Here's how the part is built. I have some questions about the finished solid (model axes, mm). A direction names the side the tool comes from. Coordinates: 2 decimals unless noted, no trailing zeros. Order: outer loops, then holes, each group sorted by start corner. A loop starts at its lowest first (then second) coordinate and runs counter-clockwise, first axis right, second up. Notation, with made-up numbers: (-3.5, 84.5) - (24.5, 84.5) arc R5 ccw to (24.5, 90.5) - close; hole circle Ø5 at (18, 15.5). An arc over 180 degrees is marked (long way). Use one line per item in the form item = value. Start each with the question number.
from build123d import *

# Parameters (mm, degrees)
SKETCH1_R                      = 16
SKETCH1_R_2                    = 4
BOSS_EXTRUDE1_DEPTH            = 2
SKETCH2_R                      = 8
SKETCH2_R_2                    = 4
BOSS_EXTRUDE2_DEPTH            = 11
M4_CLEARANCE_HOLE1_D           = 4.5
M4_CLEARANCE_HOLE1_DEPTH       = 13
M4_CLEARANCE_HOLE1_CSINK_D     = 4.55
M4_CLEARANCE_HOLE1_CSINK_ANGLE = 90
M4_CLEARANCE_HOLE1_TIP         = 1.351936393


with BuildPart() as part:
    # Sketch1 → Boss-Extrude1 (new body)
    with BuildSketch(Plane(origin=(0, 0, 0), x_dir=(1, 0, 0), z_dir=(0, 1, 0))):
        Circle(SKETCH1_R)
        Circle(SKETCH1_R_2, mode=Mode.SUBTRACT)
    extrude(amount=BOSS_EXTRUDE1_DEPTH)

    # Sketch2 → Boss-Extrude2 (add)
    with BuildSketch(Plane(origin=(0, 2, 0), x_dir=(1, 0, 0), z_dir=(0, 1, 0))):
        Circle(SKETCH2_R)
        Circle(SKETCH2_R_2, mode=Mode.SUBTRACT)
    extrude(amount=BOSS_EXTRUDE2_DEPTH)

    # M4 Clearance Hole1
    with Locations(Plane(origin=(0, 0, 0), x_dir=(-1, 0, 0), z_dir=(0, -1, 0))):
        with Locations((-8.35, 8.35), (8.35, 8.35), (8.35, -8.35), (-8.35, -8.35)):
            CounterSinkHole(M4_CLEARANCE_HOLE1_D / 2, M4_CLEARANCE_HOLE1_CSINK_D / 2, depth=M4_CLEARANCE_HOLE1_DEPTH, counter_sink_angle=M4_CLEARANCE_HOLE1_CSINK_ANGLE)
            with Locations((0, 0, -(M4_CLEARANCE_HOLE1_DEPTH + M4_CLEARANCE_HOLE1_TIP / 2))):  # 118° drill point
                Cone(0, M4_CLEARANCE_HOLE1_D / 2, M4_CLEARANCE_HOLE1_TIP, mode=Mode.SUBTRACT)


solid = part.part
1) Which directions (+Z, -Z, +X, -X, +Y, -Y) give clear straight access to the entire face, cutting with the end or side of a thin tool? Please do faces 1 (the flat face through (3, 0, 3)), 2 (the flat face through (-7.3, 2, -3.8)).
2) Suppose I cut it at D-D, the plane y = 9. List the corners of the cut face in (x, z) for me.
3) I need wall thicknesses on probe 1 along Z at (x, y) = (8.35, 0.95); probe 2 along X at (y, z) = (1.25, 9). Which ranges of each line are inside material? Lowest first, please. Write a range as [from, to].
4) Suppose I cut it at A-A, the plane z = 0. List the corners of the cut face in (x, y) for me.
5) Suppose I cut it at C-C, the plane y = 1.25. List the corners of the cut face in (x, z) for me.
6) If we mould it in two halves opening along Z, with no side actions, what happens to faces 3 (the cylindrical face through (-10.6, 1, 8.3)), 4 (the flat face through (-4, 13, 2)), 5 (the cylindrical face through (-1.73, 7.42, 7.81))? For each: pulls with the +Z half, pulls with the -Z half, needs draft (parallel to the pull), parting line crosses it, or undercut.
7) For pin 1 (1 mm diameter, centred on y = 11.5, z = -0.5, fed in from +X); pin 2 (7 mm diameter, centred on x = 8.35, z = -8.35, fed in from +Y); pin 3 (1 mm diameter, centred on x = -6, y = 1.5, fed in from -Z) (3 decimals), each with a flat end and sliding along its axis, tell me the tip position at first contact or that it passes through.
8) Suppose I cut it at B-B, the plane x = -1. List the corners of the cut face in (y, z) for me.
From the geometry:
q1.face_1 = +Z, -Z, +X, -X, -Y
q1.face_2 = +Y
q2.outline = circle Ø16 at (0, 0); hole circle Ø8 at (0, 0)
q3.probe_1 = [-13.65, -10.6], [-6.1, 6.1], [10.6, 13.65]
q3.probe_2 = [-13.23, -10.5], [-6.2, 6.2], [10.5, 13.23]
q4.outline = (-16, 0) - (-4, 0) - (-4, 13) - (-8, 13) - (-8, 2) - (-16, 2) - close; (4, 0) - (16, 0) - (16, 2) - (8, 2) - (8, 13) - (4, 13) - close
q5.outline = circle Ø32 at (0, 0); hole circle Ø4.5 at (-8.35, -8.35); hole circle Ø4.5 at (-8.35, 8.35); hole circle Ø8 at (0, 0); hole circle Ø4.5 at (8.35, -8.35); hole circle Ø4.5 at (8.35, 8.35)
q6.face_3 = undercut
q6.face_4 = needs draft
q6.face_5 = parting line crosses it
q7.pin_1 = 8
q7.pin_2 = 2
q7.pin_3 = -15.025
q8.outline = (0, -15.97) - (2, -15.97) - (2, -7.94) - (13, -7.94) - (13, -3.87) - (0, -3.87) - close; (0, 3.87) - (13, 3.87) - (13, 7.94) - (2, 7.94) - (2, 15.97) - (0, 15.97) - close
